Model file for the job. Use its own axes, mm. Face numbers are marked on the shaded views. A direction names the side the tool comes from. Coordinates: 2 decimals unless noted, no trailing zeros. Order: outer loops, then holes, each group sorted by start corner. A loop starts at its lowest first (then second) coordinate and runs counter-clockwise, first axis right, second up. Notation, with made-up numbers: (46.5, 41) -> (68.5, 41) arc R8 ccw to (68.5, 46) -> close; hole circle Ø8 at (-8.5, -8). An arc over 180 degrees is marked (long way). Return JSON: item names as keys, results as strings. Group by question number.
1) Which spindle directions (+Z, -Z, +X, -X, +Y, -Y) get a long thin tool onto all of the face, cutting with end or side? Do the marked faces 1 and 2. Say none if no direction does.
2) Probe line 1 (Y direction, x = -577, z = 257.5) (3 decimals); line 2 (X direction, y = -287.5, z = -22); line 3 (Z direction, x = -917, y = 160) (3 decimals). List the from-to ranges inside material, lowest first.
3) Cut at B-B (z = -61). Write the cut outline in (x, y) (3 decimals), and give its area (3 significant figures).
4) Flat gauge pins, fed straight in: pin 1 (4 mm diameter, centred on x = -1040.5, y = -438.5, fed in from +Z) (3 decimals); pin 2 (2 mm diameter, centred on x = -630.5, y = 107, fed in from +Z); pin 3 (4 mm diameter, centred on y = -407, z = 73, fed in from +X). Where does each tip first touch, or does it go through?
5) Cut at C-C (y = -308.5). Write the cut outline in (x, z) (1 decimal).
from build123d import *

# Parameters (mm, degrees)
F1_DEPTH = 1219.2
F2_W     = 76.2
F2_H     = 609.6
F3_DEPTH = 38.1


with BuildPart() as f1:
    # F0 (on Right) → F1 (new body)
    with BuildSketch(Plane.YZ):
        Polygon((-806.45, 327.025), (-806.45, -327.025), (806.45, -327.025), (806.45, -163.5125), (403.225, -163.5125), (403.225, 0), (0, 0), (0, 163.5125), (-403.225, 163.5125), (-403.225, 327.025), align=None)
    extrude(amount=-F1_DEPTH)

    # F2 (on face) → F3 (join)
    with BuildSketch(Plane.YZ):
        with Locations((-604.8375, 479.425)):
            Rectangle(F2_W, F2_H)
    extrude(amount=F3_DEPTH)


solid = f1.part
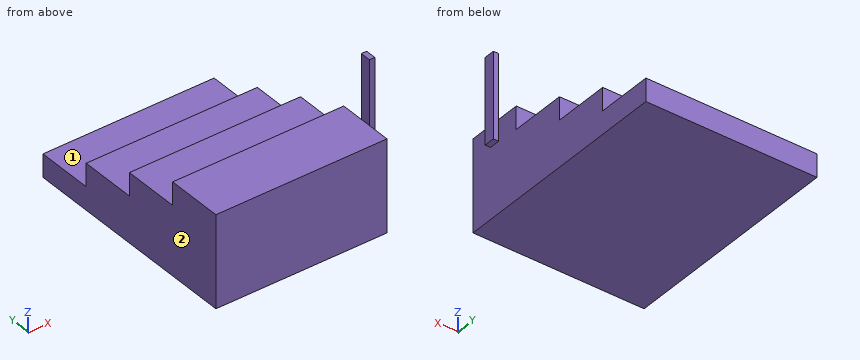
Answers below:
{
 "1": {"face 1": "+Z, +X, -X, +Y", "face 2": "+Z, -Z, -X, +Y, -Y"},
 "2": {"line 1": "y = -806.45 to -403.225", "line 2": "x = -1219.2 to 0", "line 3": "z = -327.025 to 0"},
 "3": {"outline": "(-1219.2, -806.45) -> (0, -806.45) -> (0, 403.225) -> (-1219.2, 403.225) -> close", "area": "1,470,000 mm^2"},
 "4": {"pin 1": "stops at z = 327.025", "pin 2": "stops at z = 0", "pin 3": "stops at x = 0"},
 "5": {"outline": "(-1219.2, -327) -> (0, -327) -> (0, 163.5) -> (-1219.2, 163.5) -> close"}
}
